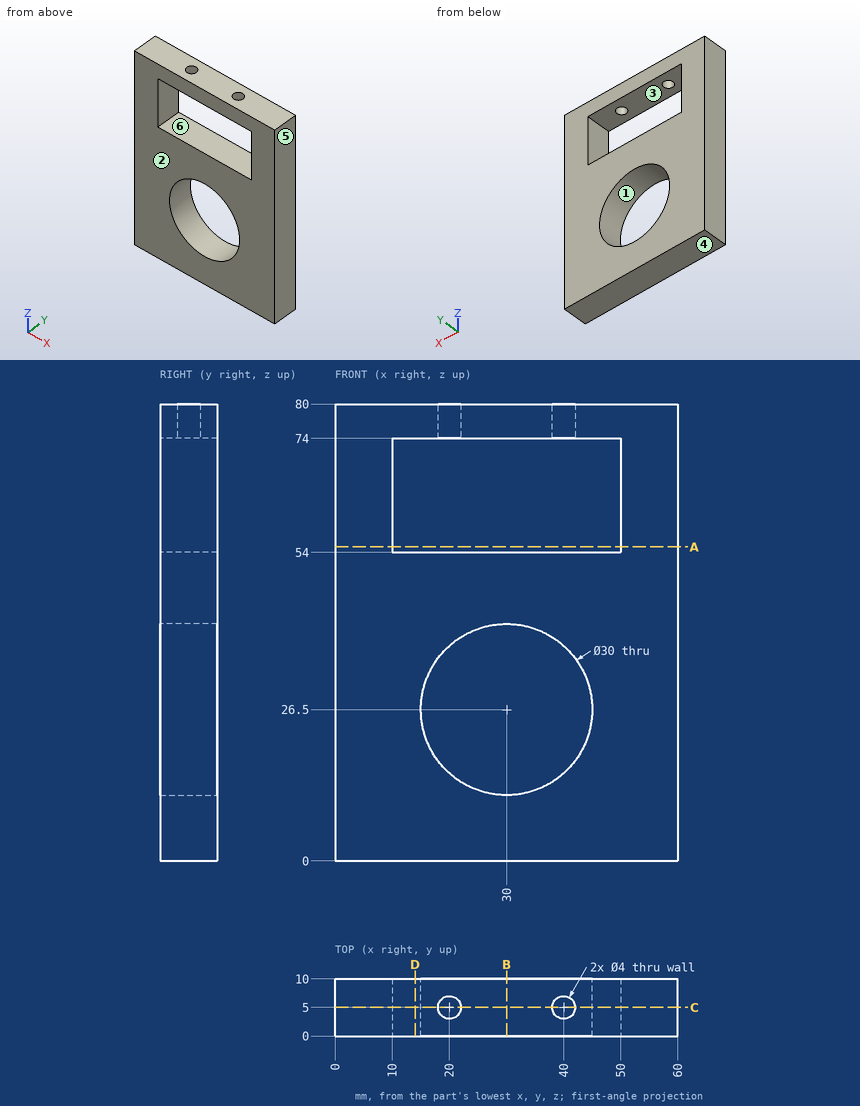
Geometry check sheet. Reference: drawing and pictorial views, mm from the part's lowest x, y, z. A direction names the side the tool comes from. Round coordinates to 2 decimals unless told otherwise and drop trailing zeros. Order: outer loops, then holes, each group sorted by start corner. A loop starts at its lowest first (then second) coordinate and runs counter-clockwise, first axis right, second up. Notation, with made-up numbers: M 54.25,66.5 L 101.25,66.5 A32 cw 101.25,95.5 Z; hole C 38.5,61.25 d6. An arc over 180 degrees is marked long. Write item = value, one per line.
Q1. Depth check by flat-ended pin: pin 1 Ø6 at (y, z) = (6.5, 21) entering from -X. Enter the tip coordinate at first touch or a pass-through.
Answer block:
pin_1 = 0
Q2. Section check A-A (z = 55). Enter the section's corners in (x, y), plus the area to 3 significant figures.
Answer block:
outline = M 0,0 L 10,0 L 10,10 L 0,10 Z; M 50,0 L 60,0 L 60,10 L 50,10 Z
area = 200 mm^2
Q3. Release check for a two-part mould opening along Z. For the marked faces 1, 2, 3 and 4 record: released by +Z, released by -Z, zero draft, split by the parting line, or undercut.
Answer block:
face_1 = undercut
face_2 = zero draft
face_3 = undercut
face_4 = released by -Z
Q4. Scan lines: line 1 (Y direction, x = 40, z = 78); line 2 (Z direction, x = 27.5, y = 6); line 3 (Z direction, x = 31.5, y = 9.5). Record each from-to range of solid material in increasing order.
Answer block:
line_1 = 0 to 3, 7 to 10
line_2 = 0 to 11.71, 41.29 to 54, 74 to 80
line_3 = 0 to 11.58, 41.42 to 54, 74 to 80
Q5. Section check D-D (x = 14). Enter the section's corners in (y, z).
Answer block:
outline = M 0,0 L 10,0 L 10,54 L 0,54 Z; M 0,74 L 10,74 L 10,80 L 0,80 Z
Q6. Section check C-C (y = 5). Enter the section's corners in (x, z).
Answer block:
outline = M 0,0 L 60,0 L 60,80 L 42,80 L 42,74 L 50,74 L 50,54 L 10,54 L 10,74 L 18,74 L 18,80 L 0,80 Z; M 22,74 L 38,74 L 38,80 L 22,80 Z; hole C 30,26.5 d30
Q7. Section check B-B (x = 30). Enter the section's corners in (y, z), plus the area to 3 significant figures.
Answer block:
outline = M 0,0 L 10,0 L 10,11.5 L 0,11.5 Z; M 0,41.5 L 10,41.5 L 10,54 L 0,54 Z; M 0,74 L 10,74 L 10,80 L 0,80 Z
area = 300 mm^2
Q8. Set-up check for the marked faces 5 and 6: record each of +Z, -Z, +X, -X, +Y, -Y from which the full face is reachable in a straight line by a thin tool's end or side.
Answer block:
face_5 = +Z, -Z, +X, +Y, -Y
face_6 = +Y, -Y
